Print and shaded views of the part. All mm, measured from the part's lowest x, y and z. A direction names the side the tool comes from. Round coordinates to 2 decimals unless told otherwise and drop trailing zeros. Order: outer loops, then holes, each group sorted by start corner. A loop starts at its lowest first (then second) coordinate and runs counter-clockwise, first axis right, second up. Notation, with made-up numbers: (-29.5, 68.25) - (21.5, 68.25) arc R26 ccw to (21.5, 85.25) - close; hole circle Ø2 at (16, 89). An arc over 180 degrees is marked (long way). Write item = value, one per line.
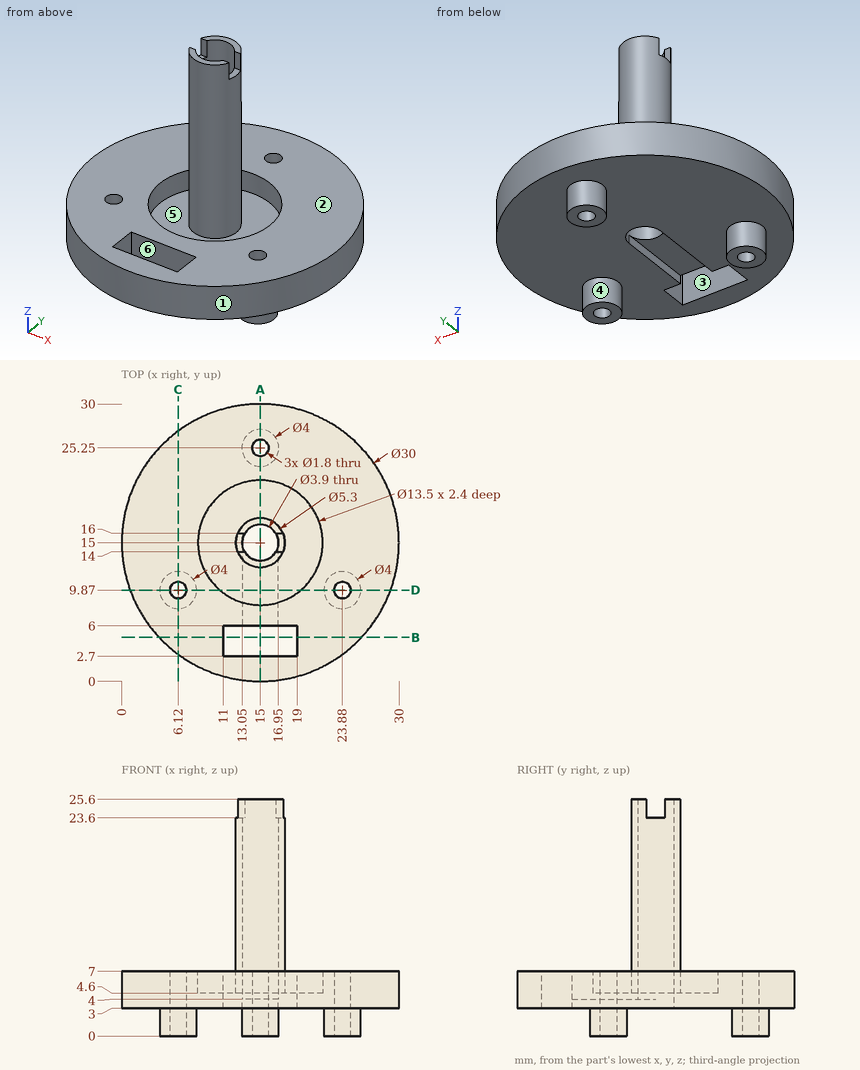
(1) Band-saw the part on D-D on y = 9.87. List the corners of the cut face in (x, z), plus the area to 3 significant figures.
Solved:
outline = (0.9, 3) - (4.12, 3) - (4.12, 0) - (5.22, 0) - (5.22, 7) - (0.9, 7) - close; (7.02, 0) - (8.12, 0) - (8.12, 3) - (13.05, 3) - (13.05, 4) - (16.95, 4) - (16.95, 3) - (21.88, 3) - (21.88, 0) - (22.98, 0) - (22.98, 7) - (19.39, 7) - (19.39, 4.6) - (10.61, 4.6) - (10.61, 7) - (7.02, 7) - close; (24.78, 0) - (25.88, 0) - (25.88, 3) - (29.1, 3) - (29.1, 7) - (24.78, 7) - close
area = 86.6 mm²
(2) Band-saw the part on A-A on x = 15. List the corners of the cut face in (y, z), plus the area to 3 significant figures.
Solved:
outline = (0, 3) - (2.7, 3) - (2.7, 7) - (0, 7) - close; (6, 4) - (13.05, 4) - (13.05, 25.6) - (12.35, 25.6) - (12.35, 4.6) - (8.25, 4.6) - (8.25, 7) - (6, 7) - close; (16.95, 3) - (23.25, 3) - (23.25, 0) - (24.35, 0) - (24.35, 7) - (21.75, 7) - (21.75, 4.6) - (17.65, 4.6) - (17.65, 25.6) - (16.95, 25.6) - close; (26.15, 0) - (27.25, 0) - (27.25, 3) - (30, 3) - (30, 7) - (26.15, 7) - close
area = 89.9 mm²
(3) Drop flat-ended pins along their axis: pin 1 (1.2 mm diameter, centred on x = 13.5, z = 5.5, fed in from +Y); pin 2 (8 mm diameter, centred on x = 23.5, z = 12, fed in from +Y); pin 3 (6 mm diameter, centred on x = 18, z = 21, fed in from +Y); pin 4 (1 mm diameter, centred on y = 5, z = 5.5, fed in from +X). Give the stop position or say it passes through.
Solved:
pin_1 = 29.97
pin_2 = through
pin_3 = 17.65
pin_4 = 26.61
(4) Pull direction X, two halves, no side cores. Call the marked faces 1, 2 and 3: released by +X, released by -X, zero draft, split by the parting line, or undercut.
Solved:
face_1 = split by the parting line
face_2 = zero draft
face_3 = undercut
(5) Probe line 1 along Y through (x, z) = (15, 4.5); line 2 along X through (y, z) = (15, 14.75); line 3 along X through (y, z) = (20.5, 5.5). List the from-to ranges inside material, lowest first.
Solved:
line_1 = 0 to 2.7, 6 to 13.05, 16.95 to 24.35, 26.15 to 30
line_2 = 12.35 to 13.05, 16.95 to 17.65
line_3 = 1.04 to 11.09, 18.91 to 28.96
(6) Band-saw the part on C-C on x = 6.12. List the corners of the cut face in (y, z).
Solved:
outline = (2.91, 3) - (7.87, 3) - (7.87, 0) - (8.97, 0) - (8.97, 7) - (2.91, 7) - close; (10.77, 0) - (11.87, 0) - (11.87, 3) - (27.09, 3) - (27.09, 7) - (10.77, 7) - close
(7) Tool access for the marked faces 4, 5 and 6: list every direction of +Z, -Z, +X, -X, +Y, -Y with a clear straight run to the whole face (end or side of a thin tool).
Solved:
face_4 = -Z
face_5 = +Z
face_6 = +Z, -Z
(8) Band-saw the part on B-B on y = 4.75. List the corners of the cut face in (x, z), plus the area to 3 significant figures.
Solved:
outline = (4.05, 3) - (11, 3) - (11, 7) - (4.05, 7) - close; (19, 3) - (25.95, 3) - (25.95, 7) - (19, 7) - close
area = 55.6 mm²
